The model under review builds one solid part; all positions refer to its coordinate system, in mm. A direction names the side the tool comes from. Give positions to 0.01 mm unless a question says otherwise; leave off trailing zeros. Loops run counter-clockwise (first coordinate to the right, second up) from the corner with the lowest first, then second, coordinate; pieces in that order, holes last. Notation, with made-up numbers: M 3.25,8 L 23.25,8 A6 cw 23.25,15 Z; hole C -34.5,51.25 d11. An arc over 180 degrees is marked long. One line per item, written item: value. Start each with the question number.
Q1. We need section D-D on z = -4.5. Write out the cut boundary in (x, y).
Q2. We need section C-C on x = -13. Write out the cut boundary in (y, z), plus the area to 3 significant figures.
Q3. Mouldability with a two-part tool opening along X and no side actions: class faces 4 (the face through (46.038, 28, 2)), 5 (the face through (-41.24, 27.5, 2.46)), 6 (the face through (-20, 0, -1)) as released by +X, released by -X, zero draft, split by the parting line, or undercut.
Q4. We need section B-B on y = 28.92. Write out the cut boundary in (x, z).
Q5. To check wall thickness, follow line 1 along Y through (x, z) = (-17.5, 3.75); line 2 along Y through (x, z) = (13, 4); line 3 along X through (y, z) = (0, 0). State the ranges of each line that lie inside material, in increasing order. Write a range as from..to.
Q6. For faces 1 (the face through (0, 10, -1)), 2 (the face through (-27, -24.5, 2)), 3 (the face through (7.5, 17, 2)), list the 3-axis set-ups (+Z, -Z, +X, -X, +Y, -Y) from which the entire face can be reached by the end or side of a thin tool; tool diameter is ignored.
Q7. We need section A-A on x = 24.5. Write out the cut boundary in (y, z).
Q8. For pin 1 (4 mm diameter, centred on x = 11.5, z = -5, fed in from -Y); pin 2 (2 mm diameter, centred on x = -1, y = -17, fed in from -Z); pin 3 (2.5 mm diameter, centred on y = -19.5, z = 1.5, fed in from +X), all flat-tipped, find the tip position at first contact; note any pin that passes through.
```python
from build123d import *

# Parameters (mm, degrees)
SKETCH_1_W          = 92.075
SKETCH_1_H          = 8
SKETCH_1_R          = 1.6
SKETCH_1_W_2        = 12.5
SKETCH_1_H_2        = 20
SKETCH_1_W_3        = 15
SKETCH_1_H_3        = 14.5
EXTRUDE_1_DEPTH     = 5
SKETCH_2_R          = 1.5
CUT_EXTRUDE_1_DEPTH = 10
SKETCH_4_W          = 40
SKETCH_4_H          = 20
SKETCH_4_R          = 1.5
EXTRUDE_3_DEPTH     = 8


with BuildPart() as part:
    # 草图1 → 凸台-拉伸1 (new body)
    # profile 1 of 7: a face of its own
    with BuildSketch(Plane.XY):
        with Locations((0, 28.5)):
            Rectangle(SKETCH_1_W, SKETCH_1_H)
        with Locations((41.9735, 28.92)):
            Circle(SKETCH_1_R, mode=Mode.SUBTRACT)
        with Locations((-41.9735, 28.92)):
            Circle(SKETCH_1_R, mode=Mode.SUBTRACT)
    # profile 2 of 7: a face of its own
    with BuildSketch(Plane.XY):
        with Locations((13.75, 0)):
            Rectangle(SKETCH_1_W_2, SKETCH_1_H_2)
    # profile 3 of 7: a face of its own
    with BuildSketch(Plane.XY):
        Rectangle(SKETCH_1_W_3, SKETCH_1_H_2)
    # profile 4 of 7: a face of its own
    with BuildSketch(Plane.XY):
        with Locations((-13.75, 0)):
            Rectangle(SKETCH_1_W_2, SKETCH_1_H_2)
    # profile 5 of 7: a face of its own
    with BuildSketch(Plane.XY):
        with Locations((0, 17.25)):
            Rectangle(SKETCH_1_W_3, SKETCH_1_H_3)
    # profile 6 of 7: a face of its own
    with BuildSketch(Plane.XY):
        with Locations((0, -28.5)):
            Rectangle(SKETCH_1_W, SKETCH_1_H)
        with Locations((-41.9735, -28.92)):
            Circle(SKETCH_1_R, mode=Mode.SUBTRACT)
        with Locations((41.9735, -28.92)):
            Circle(SKETCH_1_R, mode=Mode.SUBTRACT)
    # profile 7 of 7: a face of its own
    with BuildSketch(Plane.XY):
        with Locations((0, -17.25)):
            Rectangle(SKETCH_1_W_3, SKETCH_1_H_3)
    extrude(amount=EXTRUDE_1_DEPTH)

    # 草图2 → 切除-拉伸1 (cut)
    with BuildSketch(Plane.XY.offset(5)):
        with Locations((13, 0)):
            Circle(SKETCH_2_R)
        with Locations((-13, 0)):
            Circle(SKETCH_2_R)
    extrude(amount=-CUT_EXTRUDE_1_DEPTH, mode=Mode.SUBTRACT)

    # 草图4 → 凸台-拉伸3 (add)
    with BuildSketch(Plane(origin=(0, 0, 0), x_dir=(-1, 0, 0), z_dir=(0, 0, -1))):
        Rectangle(SKETCH_4_W, SKETCH_4_H)
        with Locations(Location((-13, 0, 0), (0, 0, 180))):
            Circle(SKETCH_4_R, mode=Mode.SUBTRACT)
        with Locations(Location((13, 0, 0), (0, 0, 180))):
            Circle(SKETCH_4_R, mode=Mode.SUBTRACT)
    extrude(amount=EXTRUDE_3_DEPTH)


solid = part.part
```
Solved:
1. outline: M -20,-10 L 20,-10 L 20,10 L -20,10 Z; hole C -13,0 d3; hole C 13,0 d3
2. outline: M -32.5,0 L -24.5,0 L -24.5,5 L -32.5,5 Z; M -10,-8 L -1.5,-8 L -1.5,5 L -10,5 Z; M 1.5,-8 L 10,-8 L 10,5 L 1.5,5 Z; M 24.5,0 L 32.5,0 L 32.5,5 L 24.5,5 Z
2. area: 301 mm2
3. face 4: released by +X
3. face 5: undercut
3. face 6: released by -X
4. outline: M -46.04,0 L -43.57,0 L -43.57,5 L -46.04,5 Z; M -40.37,0 L 40.37,0 L 40.37,5 L -40.37,5 Z; M 43.57,0 L 46.04,0 L 46.04,5 L 43.57,5 Z
5. line 1: -32.5..-24.5, -10..10, 24.5..32.5
5. line 2: -32.5..-24.5, -10..-1.5, 1.5..10, 24.5..32.5
5. line 3: -20..-14.5, -11.5..11.5, 14.5..20
6. face 1: -Z
6. face 2: +Z, -Z, -X
6. face 3: +Z, -Z, +X
7. outline: M -32.5,0 L -24.5,0 L -24.5,5 L -32.5,5 Z; M 24.5,0 L 32.5,0 L 32.5,5 L 24.5,5 Z
8. pin 1: y = -10
8. pin 2: z = 0
8. pin 3: x = 7.5
